Can you work these out from the model? Positions are in its coordinate system, mm. A direction names the side the tool comes from. Round coordinates to 2 decimals unless told otherwise and drop trailing zeros. Write each loop counter-clockwise with the first axis right and the second up, starting at its lowest first coordinate (ties: lowest second). Pieces come first, ordered by that corner, then holes. Notation, with made-up numbers: (43.25, -19.5) -> (63.25, -19.5) arc R24 ccw to (63.25, -0.5) -> close; hole circle Ø5 at (89, 15.5). An arc over 180 degrees is marked (long way). Use CSV: the item, a comma, the result in double quotes.
```python
from build123d import *

# Parameters (mm, degrees)
F0_R     = 1.4019816861
F1_DEPTH = 3


with BuildPart() as f1:
    # F0 (on Top) → F1 (new body)
    with BuildSketch(Plane.XY):
        with BuildLine():
            Line((-18.017849557, -17.3308135222), (-24.017849557, -6.9385086768))
            ThreePointArc((-24.017849557, -6.9385086768), (-21.6506350946, -12.5), (-18.017849557, -17.3308135222))
        make_face()
        with BuildLine():
            Line((0, 25), (0, 24.269322199))
            Line((0, 24.269322199), (6, 24.269322199))
            ThreePointArc((6, 24.269322199), (3.0221635482, 24.8166582659), (0, 25))
        make_face()
        with BuildLine():
            Line((-6, 24.269322199), (0, 24.269322199))
            Line((0, 24.269322199), (0, 25))
            ThreePointArc((0, 25), (-3.0221635482, 24.8166582659), (-6, 24.269322199))
        make_face()
        with BuildLine():
            Line((0, 15), (0, 5.84))
            Line((0, 5.84), (5.96, 5.84))
            Line((5.96, 5.84), (5.96, 3.4871956259))
            Line((5.96, 3.4871956259), (6, 3.4641016151))
            Line((6, 3.4641016151), (6, 13.7477270849))
            ThreePointArc((6, 13.7477270849), (3.0646446553, 14.683594694), (0, 15))
        make_face()
        with BuildLine():
            Line((-4.04, 5.84), (0, 5.84))
            Line((0, 5.84), (0, 15))
            ThreePointArc((0, 15), (-3.0646446553, 14.683594694), (-6, 13.7477270849))
            Line((-6, 13.7477270849), (-6, 3.4641016151))
            Line((-6, 3.4641016151), (-14.9058808998, -1.6777111197))
            ThreePointArc((-14.9058808998, -1.6777111197), (-12.9903810568, -7.5), (-8.9058808998, -12.0700159651))
            Line((-8.9058808998, -12.0700159651), (-4.04, -9.2606983178))
            Line((-4.04, -9.2606983178), (-4.04, 0))
            Line((-4.04, 0), (-4.04, 4.5957081427))
            Line((-4.04, 4.5957081427), (-4.04, 5.84))
        make_face()
        with BuildLine():
            ThreePointArc((-6, 13.7477270849), (-3.0646446553, 14.683594694), (0, 15))
            Line((0, 15), (0, 24.269322199))
            Line((0, 24.269322199), (-6, 24.269322199))
            Line((-6, 24.269322199), (-6, 13.7477270849))
        make_face()
        with Locations((-3, 20)):
            Circle(F0_R, mode=Mode.SUBTRACT)
        with BuildLine():
            ThreePointArc((14.9058808998, -1.6777111197), (12.9903810568, -7.5), (8.9058808998, -12.0700159651))
            Line((8.9058808998, -12.0700159651), (18.0175705244, -17.3306524227))
            Line((18.0175705244, -17.3306524227), (24.0175705244, -6.9383475773))
            Line((24.0175705244, -6.9383475773), (14.9058808998, -1.6777111197))
        make_face()
        with Locations((15.8205080757, -12.5980762114)):
            Circle(F0_R, mode=Mode.SUBTRACT)
        with Locations((18.8205080757, -7.4019237886)):
            Circle(F0_R, mode=Mode.SUBTRACT)
        with BuildLine():
            Line((-10.7937886276, -13.16), (-8.9058808998, -12.0700159651))
            ThreePointArc((-8.9058808998, -12.0700159651), (-12.9903810568, -7.5), (-14.9058808998, -1.6777111197))
            Line((-14.9058808998, -1.6777111197), (-24.017849557, -6.9385086768))
            Line((-24.017849557, -6.9385086768), (-18.017849557, -17.3308135222))
            Line((-18.017849557, -17.3308135222), (-15.6435308888, -15.96))
            Line((-15.6435308888, -15.96), (-16.04, -15.96))
            Line((-16.04, -15.96), (-16.04, -13.9827696588))
            ThreePointArc((-16.04, -13.9827696588), (-16.7309554904, -11.5319438776), (-14.4185263896, -12.5980762114))
            ThreePointArc((-14.4185263896, -12.5980762114), (-14.4482255838, -12.8851187355), (-14.5360648874, -13.16))
            Line((-14.5360648874, -13.16), (-10.7937886276, -13.16))
        make_face()
        with Locations((-18.8205080757, -7.4019237886)):
            Circle(F0_R, mode=Mode.SUBTRACT)
        with BuildLine():
            Line((0, 24.269322199), (0, 15))
            ThreePointArc((0, 15), (3.0646446553, 14.683594694), (6, 13.7477270849))
            Line((6, 13.7477270849), (6, 24.269322199))
            Line((6, 24.269322199), (0, 24.269322199))
        make_face()
        with Locations((3, 20)):
            Circle(F0_R, mode=Mode.SUBTRACT)
        with BuildLine():
            Line((6, 0), (5.96, 0))
            Line((5.96, 0), (5.96, -10.3692108346))
            Line((5.96, -10.3692108346), (8.9058808998, -12.0700159651))
            ThreePointArc((8.9058808998, -12.0700159651), (12.9903810568, -7.5), (14.9058808998, -1.6777111197))
            Line((14.9058808998, -1.6777111197), (6, 3.4641016151))
            Line((6, 3.4641016151), (6, 0))
        make_face()
        with BuildLine():
            Line((6, 13.7477270849), (6, 3.4641016151))
            Line((6, 3.4641016151), (14.9058808998, -1.6777111197))
            ThreePointArc((14.9058808998, -1.6777111197), (14.9764517409, -0.8401745364), (15, 0))
            ThreePointArc((15, 0), (12.549900398, 8.2158383626), (6, 13.7477270849))
        make_face()
        with BuildLine():
            Line((-6, 3.4641016151), (-6, 13.7477270849))
            ThreePointArc((-6, 13.7477270849), (-12.9903810568, 7.5), (-14.9058808998, -1.6777111197))
            Line((-14.9058808998, -1.6777111197), (-6, 3.4641016151))
        make_face()
        with BuildLine():
            Line((24.0175705244, -6.9383475773), (18.0175705244, -17.3306524227))
            ThreePointArc((18.0175705244, -17.3306524227), (19.9806943206, -15.025575873), (21.6506348679, -12.5000003926))
            ThreePointArc((21.6506348679, -12.5000003926), (23.0028773953, -9.7910013475), (24.0175705244, -6.9383475773))
        make_face()
        with BuildLine():
            Line((-4.04, -11.16), (-4.04, -9.2606983178))
            Line((-4.04, -9.2606983178), (-8.9058808998, -12.0700159651))
            ThreePointArc((-8.9058808998, -12.0700159651), (-8.0704738939, -12.6438701009), (-7.1982220027, -13.16))
            Line((-7.1982220027, -13.16), (-4.04, -13.16))
            Line((-4.04, -13.16), (-4.04, -11.16))
        make_face()
        with BuildLine():
            ThreePointArc((-7.1982220027, -13.16), (-8.0704738939, -12.6438701009), (-8.9058808998, -12.0700159651))
            Line((-8.9058808998, -12.0700159651), (-10.7937886276, -13.16))
            Line((-10.7937886276, -13.16), (-7.1982220027, -13.16))
        make_face()
    extrude(amount=-F1_DEPTH)


solid = f1.part
```
Q1. Please list where these lines run through material, in increasing order: probe 1 along X at (y, z) = (0.5, -1.55); probe 2 along X at (y, z) = (-11.5, -1.7); probe 3 along X at (y, z) = (19, -2.7).
Resolved:
probe 1,"x = -14.99 to -4.04, 6 to 14.99"
probe 2,"x = -22.2 to -16.69, -14.95 to -4.04, 7.92 to 14.95, 16.69 to 22.2"
probe 3,"x = -6 to -3.98, -2.02 to 2.02, 3.98 to 6"
Q2. Suppose I cut it at D-D (z = -1.55). Write out the boundary of the cut face in (x, y).
Resolved:
outline,"(-24.02, -6.94) arc R25 ccw to (-18.02, -17.33) -> (-15.64, -15.96) -> (-16.04, -15.96) -> (-16.04, -13.98) arc R1.4 cw (long way) to (-14.54, -13.16) -> (-4.04, -13.16) -> (-4.04, 5.84) -> (5.96, 5.84) -> (5.96, 3.49) -> (6, 3.46) -> (6, 0) -> (5.96, 0) -> (5.96, -10.37) -> (18.02, -17.33) arc R24.99 ccw to (24.02, -6.94) -> (14.91, -1.68) arc R15 ccw to (6, 13.75) -> (6, 24.27) arc R25 ccw to (-6, 24.27) -> (-6, 13.75) arc R15 ccw to (-14.91, -1.68) -> close; hole circle Ø2.8 at (-18.82, -7.4); hole circle Ø2.8 at (-3, 20); hole circle Ø2.8 at (3, 20); hole circle Ø2.8 at (15.82, -12.6); hole circle Ø2.8 at (18.82, -7.4)"
Q3. If we mould it in two halves opening along X, with no side actions, what happens to faces 1 (the face through (-21.69, -12.43, -1.48)), 2 (the face through (-6, 4, -3)), 3 (the face through (-16.04, -15, -1))? For each: released by +X, released by -X, zero draft, split by the parting line, or undercut.
Resolved:
face 1,"released by -X"
face 2,"zero draft"
face 3,"undercut"
Q4. Suppose I cut it at C-C (y = 1). Write out the boundary of the cut face in (x, z), and give its area (3 significant figures).
Resolved:
outline,"(-14.97, -3) -> (-4.04, -3) -> (-4.04, 0) -> (-14.97, 0) -> close; (6, -3) -> (14.97, -3) -> (14.97, 0) -> (6, 0) -> close"
area,"59.7 mm^2"
Q5. Suppose I cut it at A-A (y = 20). Write out the boundary of the cut face in (x, z), and give its area (3 significant figures).
Resolved:
outline,"(-6, -3) -> (-4.4, -3) -> (-4.4, 0) -> (-6, 0) -> close; (-1.6, -3) -> (1.6, -3) -> (1.6, 0) -> (-1.6, 0) -> close; (4.4, -3) -> (6, -3) -> (6, 0) -> (4.4, 0) -> close"
area,"19.2 mm^2"
Q6. Will these pins go through, and if not, where does the flat tip stop? P1, Ø0.9, axis at y = 1.5, z = -2, coming from the -X side; P2, Ø1.5, axis at x = 13.5, z = -1.5, coming from the -Y side; P3, Ø0.9, axis at y = 16.5, z = -2, coming from the +X side; P4, Ø3, axis at x = -13, y = 13, coming from the +Z side.
Resolved:
P1,"stops at x = -14.96"
P2,"stops at y = -15.16"
P3,"stops at x = 6"
P4,"passes through"
Q7. On a 3-axis mill with a long thin cutter (end or side, diameter ignored), from which of +Z, -Z, +X, -X, +Y, -Y can I reach the whole of each face in a straight line? I mean faces 4 (the face through (-6, 19, -1)), 5 (the face through (-16.847, -16.655, -1.479)), 6 (the face through (6, 19, -1)), 7 (the face through (-17.525, -7.939, -1.479)), 8 (the face through (-6, 4, 0)). Say none if no direction works.
Resolved:
face 4,"+Z, -Z, -X, +Y"
face 5,"+Z, -Z, -Y"
face 6,"+Z, -Z, +X, +Y"
face 7,"+Z, -Z"
face 8,"+Z, +X, -X, +Y, -Y"
Q8. Suppose I cut it at B-B (x = -19.5). Write out the boundary of the cut face in (y, z).
Resolved:
outline,"(-15.64, -3) -> (-8.63, -3) -> (-8.63, 0) -> (-15.64, 0) -> close; (-6.18, -3) -> (-4.33, -3) -> (-4.33, 0) -> (-6.18, 0) -> close"
